The listing builds one solid part. Answer for the finished solid, in the listing's coordinates (mm). A direction names the side the tool comes from. Coordinates: 2 decimals unless noted, no trailing zeros. Order: outer loops, then holes, each group sorted by start corner. A loop starts at its lowest first (then second) coordinate and runs counter-clockwise, first axis right, second up. Notation, with made-up numbers: (72.5, -39.5) -> (91.5, -39.5) arc R18 cw to (91.5, -6.5) -> close; hole circle Ø3 at (33, 65.5). An arc over 180 degrees is marked (long way). Return JSON: item names as keys, results as strings.
Autodesk Inventor part; units mm, degrees
ref_plane "YZ Plane" through (0, 0, 0) normal (1, 0, 0) x (0, 1, 0)
ref_plane "XZ Plane" through (0, 0, 0) normal (0, 1, 0) x (-1, 0, 0)
ref_plane "XY Plane" through (0, 0, 0) normal (0, 0, 1) x (1, 0, 0)
sketch "Sketch1" plane through (0, 0, 0) normal (0, 0, 1) x (1, 0, 0)
  line L0 (-56.5, -63) -> (56.5, -63)
  line L1 (56.5, -63) -> (56.5, 63)
  line L2 (56.5, 63) -> (-56.5, 63)
  line L3 (-56.5, 63) -> (-56.5, -63)
  line L4 (-56.5, -63) -> (56.5, 63) construction
  line L5 (56.5, -63) -> (-56.5, 63) construction
  line L6 (56.5, -63) -> (50.5, -63)
  line L7 (50.5, -63) -> (50.5, -60)
  line L8 (50.5, -60) -> (56.5, -60)
  line L9 (56.5, -60) -> (56.5, -63)
  line L10 (0, 63) -> (0, -63)
  line L11 (-56.5, 0) -> (56.5, 0)
  line L12 (-56.5, -63) -> (-50.5, -63)
  line L13 (-50.5, -63) -> (-50.5, -60)
  line L14 (-50.5, -60) -> (-56.5, -60)
  line L15 (-56.5, -60) -> (-56.5, -63)
  line L16 (50.5, 63) -> (50.5, 60)
  line L17 (50.5, 60) -> (56.5, 60)
  line L18 (-50.5, 63) -> (-50.5, 60)
  line L19 (-50.5, 60) -> (-56.5, 60)
  line L20 (-50.5, -60) -> (50.5, -60)
  line L21 (-50.5, 60) -> (50.5, 60)
  point P0 (0, 0)
  point P1 (-50.5, -63)
  point P2 (50.5, -63)
  point P3 (50.5, 63)
  point P4 (-50.5, 63)
  dimension "d0" = 113
  dimension "d1" = 126
  dimension "d2" = 6
  dimension "d3" = 3
extrude "Extrusion1" add sketch "Sketch1" along normal mid plane 3 contours L3 L14 L13 L0 | L3 L11 L10 L20 L14 | L3 L19 L21 L10 L11 | L7 L8 L1 L0 | L10 L11 L1 L8 L20 | L3 L2 L18 L19 | L10 L21 L17 L1 L11 | L16 L2 L1 L17
sketch "Sketch2" plane through (0, 0, 1.5) normal (0, 0, 1) x (1, 0, 0)
  circle A0 centre (-3, -35) radius 4
  line L0 (-3, 0) -> (-56.5, 0)
  line L1 (-56.5, 63) -> (-56.5, -63)
  circle A1 centre (-3, 35) radius 4
  circle A2 centre (-3, 0) radius 10.5
  line L2 (56.5, -63) -> (56.5, 63)
  line L3 (50.5, 60) -> (-50.5, 60)
  dimension "d6" = 70
  dimension "d7" = 8
  dimension "d8" = 21
  dimension "d11" = 59.5
  dimension "d12" = 60
extrude "Extrusion2" cut sketch "Sketch2" against normal blind 3
properties part number "upper support"
1. Each of these flat-tipped pins is pushed along its axis until it touches: pin 1 Ø10.5 at (x, y) = (-3, -35) entering from +Z; pin 2 Ø1.5 at (x, z) = (-17, -0.5) entering from -Y. Where does it stop, or does it pass through?
Answer block:
{"pin 1": "stops at z = 1.5", "pin 2": "stops at y = -60"}
2. Determine the mould class of faces 4 (the face through (-1, -60, 0)), 5 (the face through (50.5, -62, 0)), 6 (the face through (56.5, -1, 0)), 7 (the face through (-53, 63, 0)) for opening direction X: pulls with the +X half, pulls with the -X half, needs draft (parallel to the pull), parting line crosses it, or undercut.
Answer block:
{"face 4": "undercut", "face 5": "undercut", "face 6": "pulls with the +X half", "face 7": "needs draft"}
3. The part is cut by section A-A on y = 0. Give the vertices of the cut face in (x, z).
Answer block:
{"outline": "(-56.5, -1.5) -> (-13.5, -1.5) -> (-13.5, 1.5) -> (-56.5, 1.5) -> close; (7.5, -1.5) -> (56.5, -1.5) -> (56.5, 1.5) -> (7.5, 1.5) -> close"}
4. The part is cut by section D-D on y = 35. Give the vertices of the cut face in (x, z), and give its area (3 significant figures).
Answer block:
{"outline": "(-56.5, -1.5) -> (-7, -1.5) -> (-7, 1.5) -> (-56.5, 1.5) -> close; (1, -1.5) -> (56.5, -1.5) -> (56.5, 1.5) -> (1, 1.5) -> close", "area": "315 mm2"}
5. The part is cut by section C-C on z = -0.5. Give the vertices of the cut face in (x, y).
Answer block:
{"outline": "(-56.5, -63) -> (-50.5, -63) -> (-50.5, -60) -> (50.5, -60) -> (50.5, -63) -> (56.5, -63) -> (56.5, 63) -> (50.5, 63) -> (50.5, 60) -> (-50.5, 60) -> (-50.5, 63) -> (-56.5, 63) -> close; hole circle Ø21 at (-3, 0); hole circle Ø8 at (-3, -35); hole circle Ø8 at (-3, 35)"}
6. The part is cut by section B-B on x = -3. Give the vertices of the cut face in (y, z).
Answer block:
{"outline": "(-60, -1.5) -> (-39, -1.5) -> (-39, 1.5) -> (-60, 1.5) -> close; (-31, -1.5) -> (-10.5, -1.5) -> (-10.5, 1.5) -> (-31, 1.5) -> close; (10.5, -1.5) -> (31, -1.5) -> (31, 1.5) -> (10.5, 1.5) -> close; (39, -1.5) -> (60, -1.5) -> (60, 1.5) -> (39, 1.5) -> close"}
7. Consider line 1 (Y direction, x = -3, z = 0.6); line 2 (X direction, y = 0, z = 0.85); line 3 (Y direction, x = -18.5, z = -1.2). Determine where each line is inside the solid, lowest interval first. Write a range as from..to.
Answer block:
{"line 1": "y = -60..-39, -31..-10.5, 10.5..31, 39..60", "line 2": "x = -56.5..-13.5, 7.5..56.5", "line 3": "y = -60..60"}
8. For faces 1 (the face through (53, -63, 0)), 2 (the face through (-50.5, -62, 0)), 3 (the face through (-1, 60, 0)), determine the directions among +Z, -Z, +X, -X, +Y, -Y from which every point of the face is accessible in a straight line to the end or side of a thin tool.
Answer block:
{"face 1": "+Z, -Z, +X, -X, -Y", "face 2": "+Z, -Z, -Y", "face 3": "+Z, -Z, +Y"}
